Answer from the drawing. Dimensions are ordinates in mm from the lowest x, y and z of the part. Coordinates: 2 decimals unless noted, no trailing zeros. Order: outer loops, then holes, each group sorted by start corner. A loop starts at its lowest first (then second) coordinate and runs counter-clockwise, first axis right, second up.
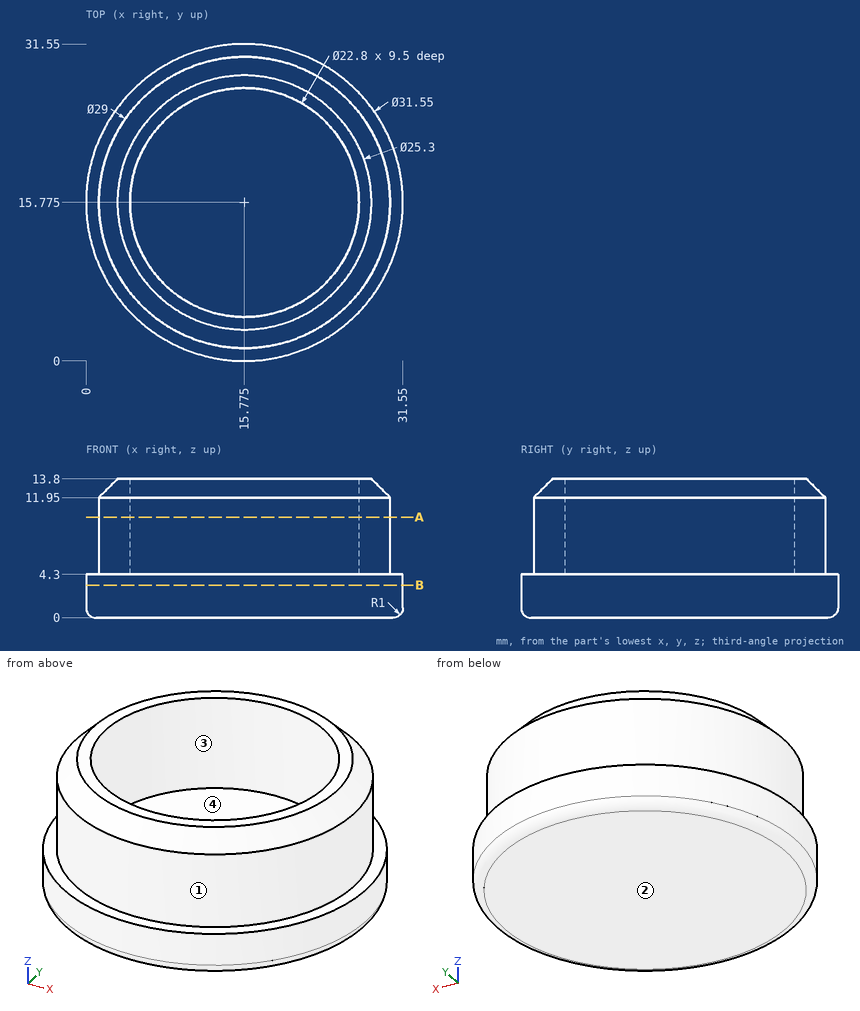
1. Consider probe 1 along X at (y, z) = (13.5, 7.75); probe 2 along X at (y, z) = (13, 10.75); probe 3 along Z at (x, y) = (25, 22). Determine where each line is inside the solid, lowest interval first.
2. The part is cut by section A-A (z = 10). Determine the outline of the cut face in (x, y) (3 decimals), plus the area to 3 significant figures.
3. The mould has two halves that part along X. Classify the marked faces 1, 2, 3 and 4: released by +X, released by -X, zero draft, split by the parting line, or undercut.
4. Flat-ended cylindrical pins translate along their axes: pin 1 (5 mm diameter, centred on y = 4.5, z = 3.5, fed in from +X); pin 2 (8 mm diameter, centred on x = 7, z = 3, fed in from +Y); pin 3 (1.5 mm diameter, centred on x = 16.5, z = 10.5, fed in from +Y) (3 decimals). Find the tip coordinate at first contact, or state that the pin passes through.
5. The part is cut by section B-B (z = 3.25). Determine the outline of the cut face in (x, y) (3 decimals), plus the area to 3 significant figures.
Worked out:
1. probe 1: x = 1.45 to 4.6, 26.95 to 30.1
1. probe 2: x = 1.54 to 4.72, 26.83 to 30.01
1. probe 3: z = 0 to 4.3
2. outline: circle Ø29 at (15.775, 15.775); hole circle Ø22.8 at (15.775, 15.775)
2. area: 252 mm2
3. face 1: split by the parting line
3. face 2: zero draft
3. face 3: undercut
3. face 4: undercut
4. pin 1: stops at x = 28.88
4. pin 2: stops at y = 30.81
4. pin 3: stops at y = 30.275
5. outline: circle Ø31.55 at (15.775, 15.775)
5. area: 782 mm2
